Design review of the part built by this model. Coordinates are the model's own, in mm. A direction names the side the tool comes from. Round coordinates to 2 decimals unless told otherwise and drop trailing zeros. Write each loop counter-clockwise with the first axis right and the second up, starting at its lowest first coordinate (ties: lowest second). Pieces come first, ordered by that corner, then holes.
from build123d import *

# Parameters (mm, degrees)
SKETCH5_R           = 3.175
BOSS_EXTRUDE3_DEPTH = 51.59375
BOSS_EXTRUDE4_DEPTH = 4.365625
SKETCH8_OUTSIDE_W   = 224.338
SKETCH8_OUTSIDE_H   = 226.058
SKETCH8_OUTSIDE_R   = 5.55625
CUT_EXTRUDE3_DEPTH  = 57.599347315
CUT_EXTRUDE3_DRAFT  = -60


with BuildPart() as part:
    # Sketch5 → Boss-Extrude3 (new body)
    with BuildSketch(Plane(origin=(27.9796875, 0, 0), x_dir=(0, 0, -1), z_dir=(1, 0, 0))):
        Circle(SKETCH5_R)
    extrude(amount=-BOSS_EXTRUDE3_DEPTH)

    # Sketch6 → Boss-Extrude4 (add)
    with BuildSketch(Plane.ZY.offset(23.6140625)):
        Polygon((5.55625, 3.207902433), (0, 6.415804866), (-5.55625, 3.207902433), (-5.55625, -3.207902433), (0, -6.415804866), (5.55625, -3.207902433), align=None)
    extrude(amount=BOSS_EXTRUDE4_DEPTH)


with BuildPart() as cut_extrude3_tool:
    # Sketch8 outside → Cut-Extrude3 (with draft: the straight prism first)
    with BuildSketch(Plane.ZY.offset(27.9796875)):
        Rectangle(SKETCH8_OUTSIDE_W, SKETCH8_OUTSIDE_H)
        Circle(SKETCH8_OUTSIDE_R, mode=Mode.SUBTRACT)
    extrude(amount=-CUT_EXTRUDE3_DEPTH)
    # Cut-Extrude3: the draft: its side faces are tilted about the plane it starts from
    cut_extrude3_sides = [cut_extrude3_tool.faces().sort_by_distance(p)[0] for p in [
        (0.819986158, -113.029, 0),
        (0.819986158, 0, 112.169),
        (0.819986158, 113.029, 0),
        (0.819986158, 0, -112.169),
        (0.819986158, 0, -5.55625),
    ]]
    draft(cut_extrude3_sides, Plane.ZY.offset(27.9796875), CUT_EXTRUDE3_DRAFT)


with BuildPart() as part_1:
    add(part.part)

    # Cut-Extrude3: cut by cut_extrude3_tool
    add(cut_extrude3_tool.part, mode=Mode.SUBTRACT)


solid = part_1.part
1) For faces 1 (the face through (2.54, -3.1, 0.69)), 2 (the face through (27.98, 0, 0)), list the 3-axis set-ups (+Z, -Z, +X, -X, +Y, -Y) from which the entire face can be reached by the end or side of a thin tool; tool diameter is ignored.
2) Add section A-A on x = 23. State the section outline as (y, z) points (3 decimals), and give its area (3 significant figures).
3) For P1, Ø3, axis at x = 5, z = -0.5, coming from the +Y side (3 decimals); P2, Ø5, axis at x = 8, z = -1.5, coming from the -Y side (3 decimals); P3, Ø5, axis at x = 15.5, y = -1, coming from the +Z side (3 decimals), all flat-tipped, find the tip position at first contact; note any pin that passes through.
4) For line 1 along X through (y, z) = (-3, 1.75); line 2 along Y through (x, z) = (23, 0) (3 decimals); line 3 along Z through (x, y) = (21.5, -0.25), list the stretches that pass through material, from the lowest coordinate up.
Computed:
1. face 1: +X
1. face 2: +Z, -Z, +X, +Y, -Y
2. outline: circle Ø6.35 at (0, 0)
2. area: 31.7 mm2
3. P1: stops at y = 3.175
3. P2: stops at y = -3.175
3. P3: stops at z = 3.175
4. line 1: x = -27.98 to -23.61
4. line 2: y = -3.175 to 3.175
4. line 3: z = -3.17 to 3.17
